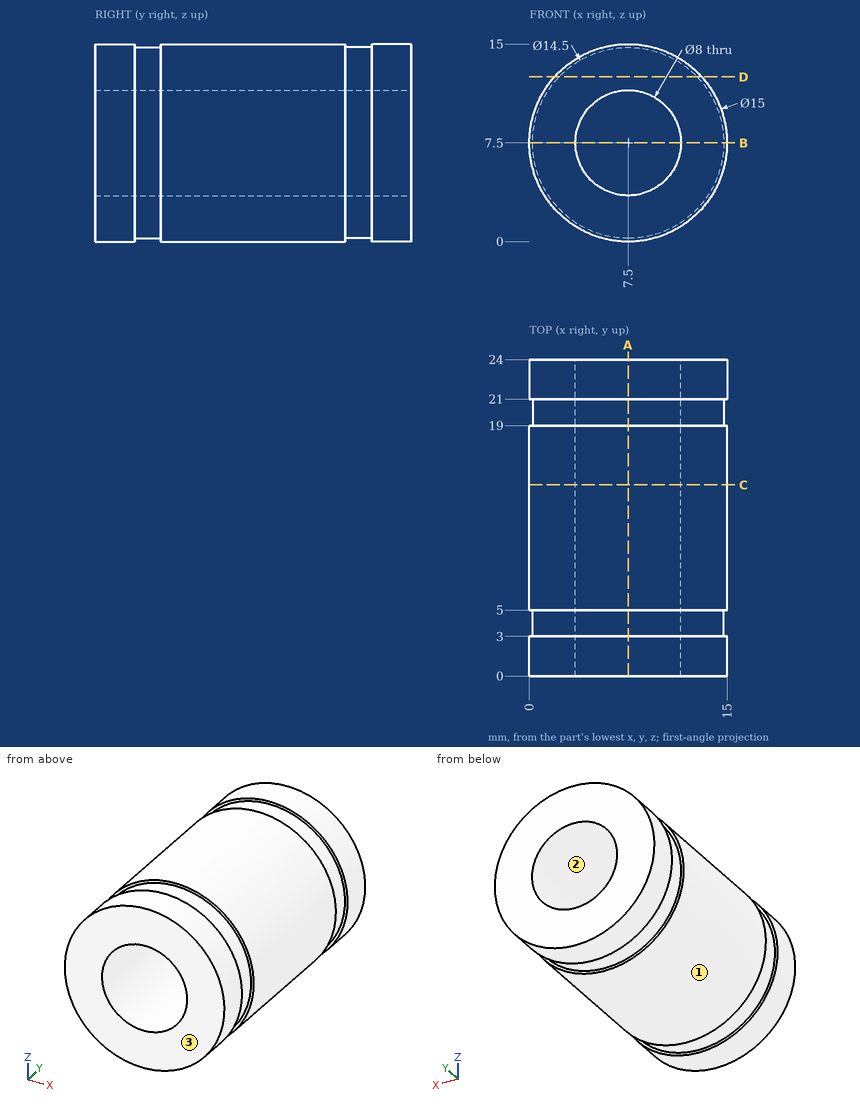
Design review of the part shown in the three views and the two pictorial views. Dimensions are in mm from the part's minimum x, y and z. Give positions to 0.01 mm unless a question says otherwise; leave off trailing zeros. Loops run counter-clockwise (first coordinate to the right, second up) from the corner with the lowest first, then second, coordinate; pieces in that order, holes last. Notation, with made-up numbers: (80, -30) -> (94, -30) arc R30 cw to (94, 0) -> close; hole circle Ø10 at (6, 39). An arc over 180 degrees is marked (long way). One line per item, written item: value.
Q1. For L1, parallel to X at y = 11.5, z = 7.5; L2, parallel to Z at x = 8.75, y = 16.25; L3, parallel to X at y = 13.5, z = 8.5, list the stretches that pass through material, from the lowest coordinate up.
Numbers:
L1: x = 0 to 3.5, 11.5 to 15
L2: z = 0.1 to 3.7, 11.3 to 14.9
L3: x = 0.07 to 3.63, 11.37 to 14.93
Q2. For pin 1 Ø4.5 at (x, z) = (10.5, 7.5) entering from -Y; pin 2 Ø1 at (y, z) = (17, 9.5) entering from -X; pin 3 Ø3 at (y, z) = (15.5, 9.5) entering from +X; pin 4 Ø5 at (y, z) = (9.5, 4.5) entering from -X, all flat-tipped, find the tip position at first contact; note any pin that passes through.
Numbers:
pin 1: stops at y = 0
pin 2: stops at x = 0.15
pin 3: stops at x = 14.98
pin 4: stops at x = 0.02
Q3. Draft analysis for pull direction Z (two halves, no side actions). For the marked faces 1, 2 and 3, state which applies: pulls with the +Z half, pulls with the -Z half, needs draft (parallel to the pull), parting line crosses it, or undercut.
Numbers:
face 1: parting line crosses it
face 2: undercut
face 3: needs draft
Q4. We need section C-C on y = 14.5. Give the boundary of the cut face in (x, z).
Numbers:
outline: circle Ø15 at (7.5, 7.5); hole circle Ø8 at (7.5, 7.5)
Q5. We need section A-A on x = 7.5. Give the boundary of the cut face in (y, z), and give its area (3 significant figures).
Numbers:
outline: (0, 0) -> (3, 0) -> (3, 0.25) -> (5, 0.25) -> (5, 0) -> (19, 0) -> (19, 0.25) -> (21, 0.25) -> (21, 0) -> (24, 0) -> (24, 3.5) -> (0, 3.5) -> close; (0, 11.5) -> (24, 11.5) -> (24, 15) -> (21, 15) -> (21, 14.75) -> (19, 14.75) -> (19, 15) -> (5, 15) -> (5, 14.75) -> (3, 14.75) -> (3, 15) -> (0, 15) -> close
area: 166 mm^2
Q6. We need section D-D on z = 12.5. Give the boundary of the cut face in (x, y).
Numbers:
outline: (1.91, 0) -> (13.09, 0) -> (13.09, 3) -> (12.75, 3) -> (12.75, 5) -> (13.09, 5) -> (13.09, 19) -> (12.75, 19) -> (12.75, 21) -> (13.09, 21) -> (13.09, 24) -> (1.91, 24) -> (1.91, 21) -> (2.25, 21) -> (2.25, 19) -> (1.91, 19) -> (1.91, 5) -> (2.25, 5) -> (2.25, 3) -> (1.91, 3) -> close
Q7. We need section B-B on z = 7.5. Give the boundary of the cut face in (x, y), and give its area (3 significant figures).
Numbers:
outline: (0, 0) -> (3.5, 0) -> (3.5, 24) -> (0, 24) -> (0, 21) -> (0.25, 21) -> (0.25, 19) -> (0, 19) -> (0, 5) -> (0.25, 5) -> (0.25, 3) -> (0, 3) -> close; (11.5, 0) -> (15, 0) -> (15, 3) -> (14.75, 3) -> (14.75, 5) -> (15, 5) -> (15, 19) -> (14.75, 19) -> (14.75, 21) -> (15, 21) -> (15, 24) -> (11.5, 24) -> close
area: 166 mm^2
